```python
from build123d import *

# Parameters (mm, degrees)
SKETCH1_R           = 5
BOSS_EXTRUDE1_DEPTH = 1.75
FILLET1_R           = 0.3


with BuildPart() as part:
    # Sketch1 → Boss-Extrude1 (new, symmetric)
    with BuildSketch(Plane.XY):
        with BuildLine():
            Line((9, -12), (-9, -12))
            ThreePointArc((-9, -12), (-11.121320344, -11.121320344), (-12, -9))
            Line((-12, -9), (-12, 9))
            ThreePointArc((-12, 9), (-11.121320344, 11.121320344), (-9, 12))
            Line((-9, 12), (9, 12))
            ThreePointArc((9, 12), (11.121320344, 11.121320344), (12, 9))
            Line((12, 9), (12, -9))
            ThreePointArc((12, -9), (11.121320344, -11.121320344), (9, -12))
        make_face()
        Circle(SKETCH1_R, mode=Mode.SUBTRACT)
    extrude(amount=BOSS_EXTRUDE1_DEPTH, both=True)

    # Fillet1
    fillet1_edges = [part.edges().sort_by_distance(p)[0] for p in [
        (0, 12, -1.75),
        (11.121320344, 11.121320344, -1.75),
        (12, 0, -1.75),
        (11.121320344, -11.121320344, -1.75),
        (11.121320344, 11.121320344, 1.75),
        (0, 12, 1.75),
        (-11.121320344, 11.121320344, 1.75),
        (-12, 0, 1.75),
        (-11.121320344, -11.121320344, 1.75),
        (0, -12, 1.75),
        (11.121320344, -11.121320344, 1.75),
        (0, -12, -1.75),
        (12, 0, 1.75),
        (-11.121320344, -11.121320344, -1.75),
        (-12, 0, -1.75),
        (-11.121320344, 11.121320344, -1.75),
    ]]
    fillet(fillet1_edges, radius=FILLET1_R)


solid = part.part
```
Check sheet for the modelled part. Datum: model origin and axes. Units: mm. Give positions to 0.01 mm unless a question says otherwise; leave off trailing zeros. Write each loop counter-clockwise with the first axis right and the second up, starting at its lowest first coordinate (ties: lowest second). Pieces come first, ordered by that corner, then holes.
Item 1: Scan lines: L1, parallel to Y at x = 0, z = 0.7; L2, parallel to X at y = -1.75, z = 1.5; L3, parallel to X at y = -8.5, z = 1.5. Record each from-to range of solid material in increasing order.
Item 2: Cross-section at C-C (z = -0.75). Enter the section's corners in (x, y), and give its area (3 significant figures).
Item 3: Cross-section at A-A (y = 0). Enter the section's corners in (x, z), and give its area (3 significant figures).
Item 4: Draft check along Z on faces 1 (the face through (-12, 0, 0)), 2 (the face through (0.2, 5.4, 1.75)), 3 (the face through (0.2, 5.4, -1.75)). Enter one of: released by +Z, released by -Z, zero draft, split by the parting line, or undercut.
Report:
1. L1: y = -12 to -5, 5 to 12
1. L2: x = -12 to -4.68, 4.68 to 12
1. L3: x = -12 to 12
2. outline: (-12, -9) arc R3 ccw to (-9, -12) - (9, -12) arc R3 ccw to (12, -9) - (12, 9) arc R3 ccw to (9, 12) - (-9, 12) arc R3 ccw to (-12, 9) - close; hole circle Ø10 at (0, 0)
2. area: 490 mm2
3. outline: (-12, -1.45) arc R0.3 ccw to (-11.7, -1.75) - (-5, -1.75) - (-5, 1.75) - (-11.7, 1.75) arc R0.3 ccw to (-12, 1.45) - close; (5, -1.75) - (11.7, -1.75) arc R0.3 ccw to (12, -1.45) - (12, 1.45) arc R0.3 ccw to (11.7, 1.75) - (5, 1.75) - close
3. area: 48.9 mm2
4. face 1: zero draft
4. face 2: released by +Z
4. face 3: released by -Z
